The drawing under review shows one solid part. Ordinate dimensions are in mm from its lowest x, y, z. A direction names the side the tool comes from. Give positions to 0.01 mm unless a question says otherwise; leave off trailing zeros. Loops run counter-clockwise (first coordinate to the right, second up) from the corner with the lowest first, then second, coordinate; pieces in that order, holes last. Notation, with made-up numbers: (-40, 57.5) -> (6, 57.5) arc R10 ccw to (6, 67.5) -> close; hole circle Ø1 at (13.25, 55). An arc over 180 degrees is marked (long way). Answer in a Markdown table with one row per item. Add a question column.
(1) Consider section B-B on y = 1.9. Write out the cut boundary in (x, z) (1 decimal).
(2) Consider section D-D on x = 14.25. Write out the cut boundary in (y, z), then the cut area to 3 significant figures.
(3) Consider section A-A on z = 8. Write out the cut boundary in (x, y) (1 decimal).
(4) Draft analysis for pull direction X (two halves, no side actions). For the marked faces 4, 5 and 6, state which applies: +X half, -X half, draft (parallel to the pull), parting line (faces both ways), or undercut.
(5) For pin 1 (1 mm diameter, centred on x = 6.5, y = 1.5, fed in from +Z); pin 2 (0.8 mm diameter, centred on x = 11.5, y = 1.5, fed in from -Z), all flat-tipped, find the tip position at first contact; note any pin that passes through.
(6) Consider section C-C on x = 20. Write out the cut boundary in (y, z).
(7) For the marked faces 1, 2 and 3, list the 3-axis set-ups (+Z, -Z, +X, -X, +Y, -Y) from which the entire face can be reached by the end or side of a thin tool; tool diameter is ignored.
(8) For line 1 (X direction, y = 0.7, z = 5.75) (1 decimal); line 2 (Z direction, x = 15.75, y = 1.35); line 3 (Z direction, x = 1.5, y = 1.25), list the stretches that pass through material, from the lowest coordinate up.
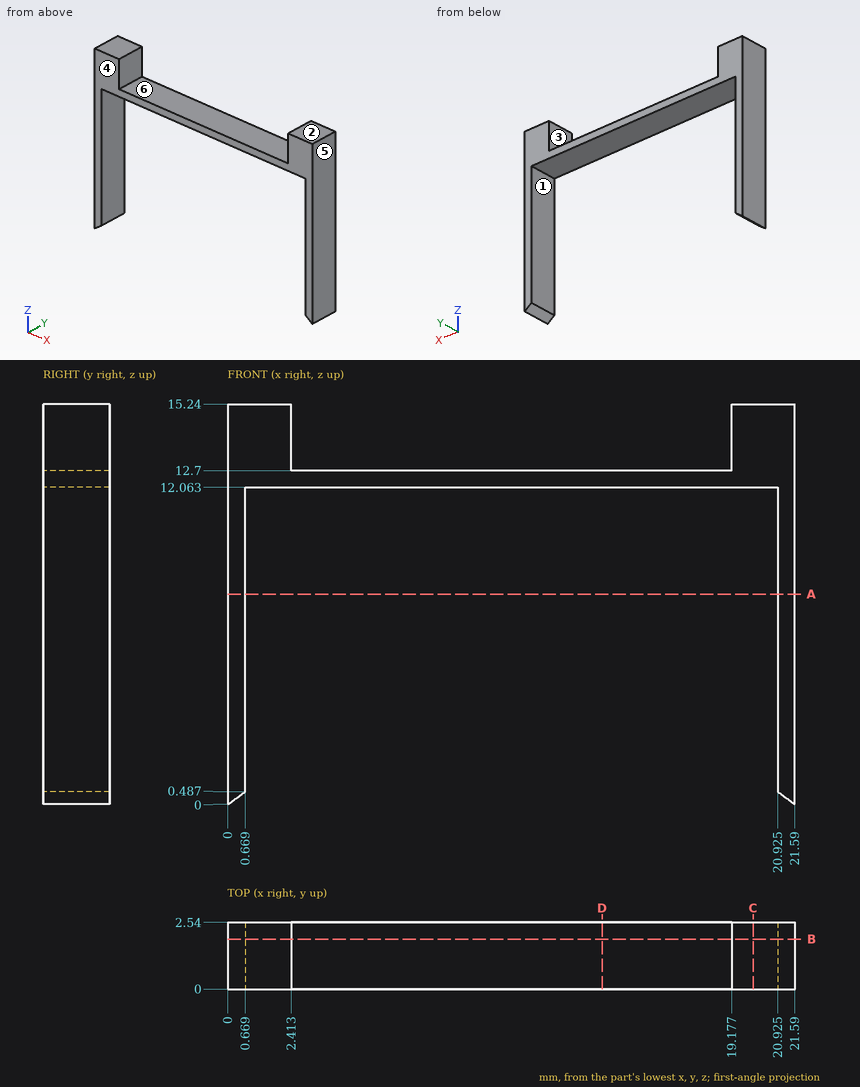
Values follow:
| question | item | result |
|---|---|---|
| 1 | outline | (0, 0) -> (0.7, 0.5) -> (0.7, 12.1) -> (20.9, 12.1) -> (20.9, 0.5) -> (21.6, 0) -> (21.6, 15.2) -> (19.2, 15.2) -> (19.2, 12.7) -> (2.4, 12.7) -> (2.4, 15.2) -> (0, 15.2) -> close |
| 2 | outline | (0, 12.06) -> (2.54, 12.06) -> (2.54, 12.7) -> (0, 12.7) -> close |
| 2 | area | 1.62 mm2 |
| 3 | outline | (0, 0) -> (0.7, 0) -> (0.7, 2.5) -> (0, 2.5) -> close; (20.9, 0) -> (21.6, 0) -> (21.6, 2.5) -> (20.9, 2.5) -> close |
| 4 | face 4 | draft |
| 4 | face 5 | +X half |
| 4 | face 6 | undercut |
| 5 | pin 1 | z = 12.7 |
| 5 | pin 2 | z = 12.06 |
| 6 | outline | (0, 12.06) -> (2.54, 12.06) -> (2.54, 15.24) -> (0, 15.24) -> close |
| 7 | face 1 | -Z, +Y, -Y |
| 7 | face 2 | +Z, +X, -X, +Y, -Y |
| 7 | face 3 | +Z, +Y, -Y |
| 8 | line 1 | 0 to 0.7, 20.9 to 21.6 |
| 8 | line 2 | 12.06 to 12.7 |
| 8 | line 3 | 12.06 to 15.24 |
